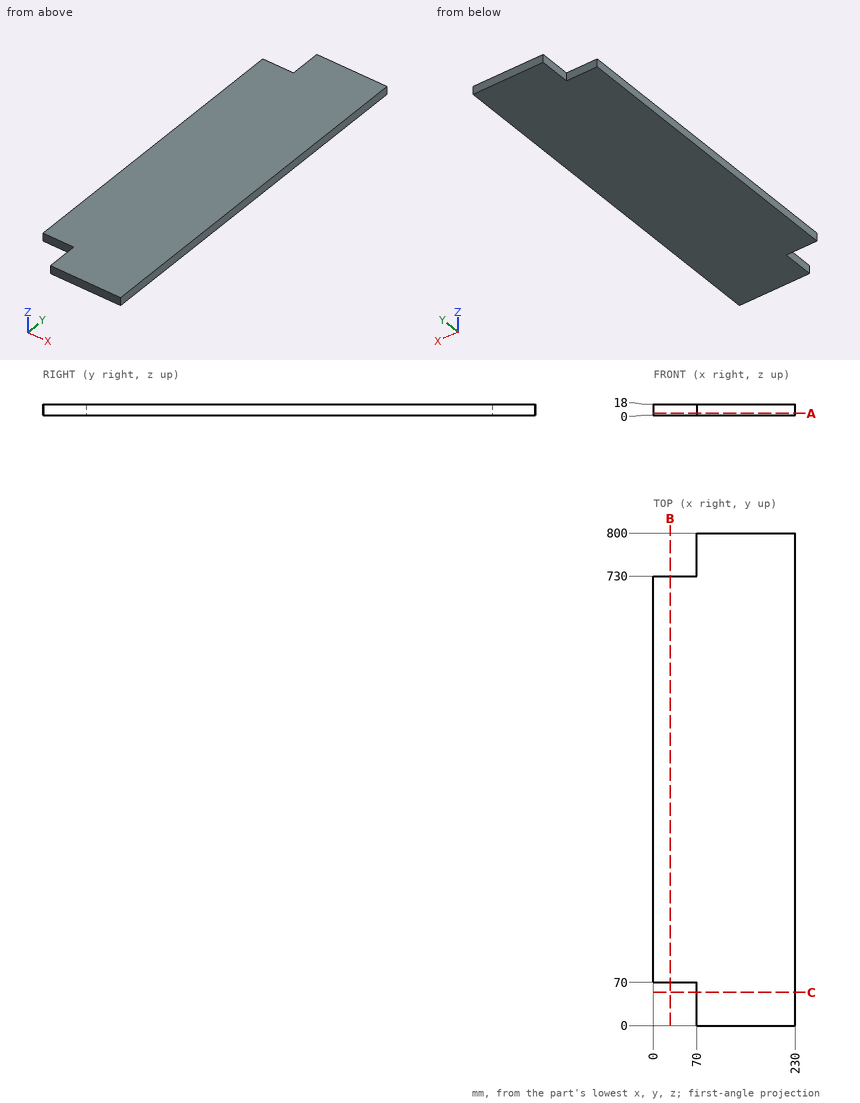
The figure shows three views and two pictorial views of one solid part (mm, origin at its lowest corner). Answer the questions. Coordinates: 2 decimals unless noted, no trailing zeros. Loops run counter-clockwise (first coordinate to the right, second up) from the corner with the lowest first, then second, coordinate; pieces in that order, holes last.
1) Find section C-C on y = 54. Write down the section's boundary in (x, z), then the cut area to 3 significant figures.
2) Find the intervals of material crossed by L1, parallel to Y at x = 10, z = 13, in increasing order.
3) Flat-ended cylindrical pins translate along their axes: pin 1 Ø9 at (x, z) = (24.5, 11) entering from +Y; pin 2 Ø6 at (y, z) = (305.5, 4.5) entering from -X; pin 3 Ø9 at (y, z) = (781, 10.5) entering from -X. Find the tip coordinate at first contact, or state that the pin passes through.
4) Find section B-B on x = 27. Write down the section's boundary in (y, z).
5) Find section A-A on z = 2.75. Write down the section's boundary in (x, y), then the cut area to 3 significant figures.
Values:
1. outline: (70, 0) - (230, 0) - (230, 18) - (70, 18) - close
1. area: 2,880 mm2
2. L1: y = 70 to 730
3. pin 1: stops at y = 730
3. pin 2: stops at x = 0
3. pin 3: stops at x = 70
4. outline: (70, 0) - (730, 0) - (730, 18) - (70, 18) - close
5. outline: (0, 70) - (70, 70) - (70, 0) - (230, 0) - (230, 800) - (70, 800) - (70, 730) - (0, 730) - close
5. area: 174,000 mm2
